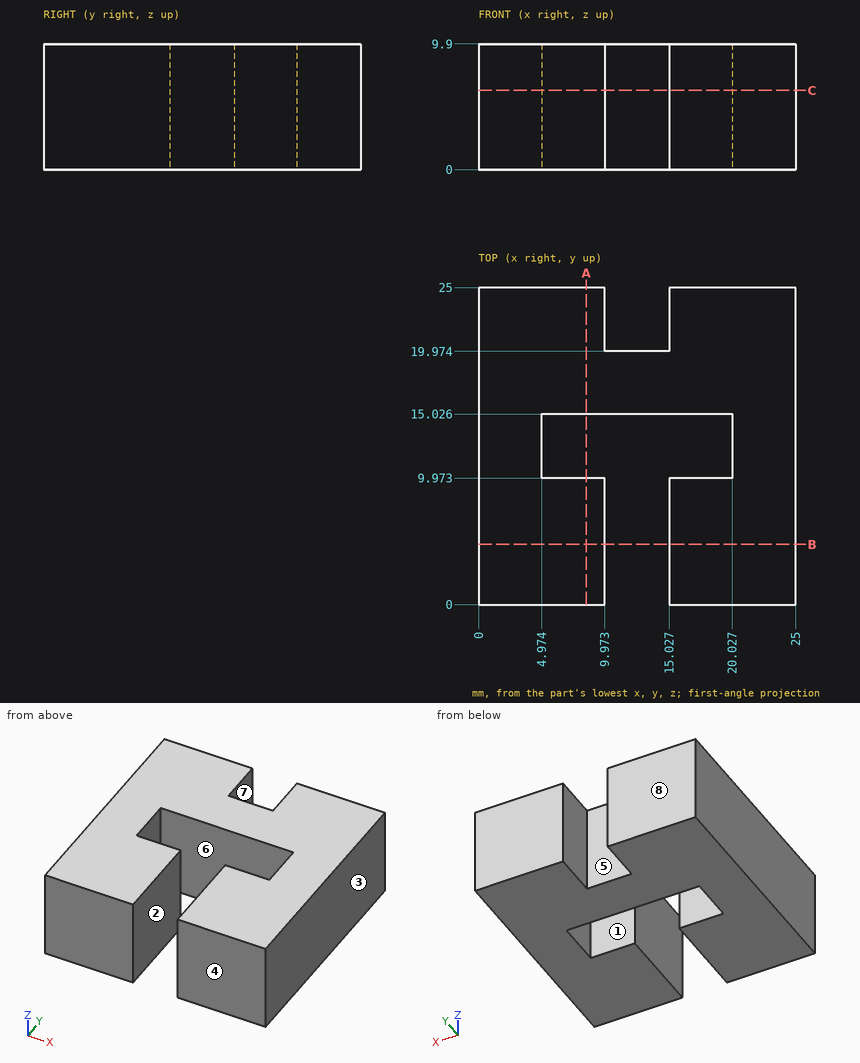
Design review of the part shown in the three views and the two pictorial views. Dimensions are in mm from the part's minimum x, y and z. A direction names the side the tool comes from. Give positions to 0.01 mm unless a question says otherwise; leave off trailing zeros. Write each loop counter-clockwise with the first axis right and the second up, starting at its lowest first coordinate (ties: lowest second). Pieces come first, ordered by that corner, then holes. Notation, with made-up numbers: M 84.5,61 L 127.5,61 A10 cw 127.5,75 Z; hole C -19,52.25 d7. An arc over 180 degrees is marked long. Answer in a Markdown table with one row per item.
Item 1: Draft analysis for pull direction Y (two halves, no side actions). For the marked faces 6, 7 and 8, state which applies: +Y half, -Y half, draft (parallel to the pull), parting line (faces both ways), or undercut.
Check sheet entries:
| item | result |
|---|---|
| face 6 | undercut |
| face 7 | draft |
| face 8 | +Y half |
Item 2: For line 1 along X through (y, z) = (12.75, 5.25) (1 decimal); line 2 along Y through (x, z) = (8, 9), list the stretches that pass through material, from the lowest coordinate up.
Check sheet entries:
| item | result |
|---|---|
| line 1 | 0 to 5, 20 to 25 |
| line 2 | 0 to 9.97, 15.03 to 25 |
Item 3: Add section A-A on x = 8.5. Give the boundary of the cut face in (y, z).
Check sheet entries:
| item | result |
|---|---|
| outline | M 0,0 L 9.97,0 L 9.97,9.9 L 0,9.9 Z; M 15.03,0 L 25,0 L 25,9.9 L 15.03,9.9 Z |
Item 4: For P1, Ø1.5, axis at y = 22.5, z = 3, coming from the -X side; P2, Ø2.5, axis at x = 12.5, z = 4.5, coming from the +Y side, all flat-tipped, find the tip position at first contact; note any pin that passes through.
Check sheet entries:
| item | result |
|---|---|
| P1 | x = 0 |
| P2 | y = 19.97 |
Item 5: Add section C-C on z = 6.25. Give the boundary of the cut face in (x, y) (1 decimal).
Check sheet entries:
| item | result |
|---|---|
| outline | M 0,0 L 10,0 L 10,10 L 5,10 L 5,15 L 20,15 L 20,10 L 15,10 L 15,0 L 25,0 L 25,25 L 15,25 L 15,20 L 10,20 L 10,25 L 0,25 Z |
Item 6: Tool access review of the marked faces 1, 2, 3, 4 and 5: name each direction out of +Z, -Z, +X, -X, +Y, -Y from which nothing blocks a thin tool from reaching the whole face with its end or side.
Check sheet entries:
| item | result |
|---|---|
| face 1 | +Z, -Z |
| face 2 | +Z, -Z, -Y |
| face 3 | +Z, -Z, +X, +Y, -Y |
| face 4 | +Z, -Z, +X, -X, -Y |
| face 5 | +Z, -Z, +Y |
